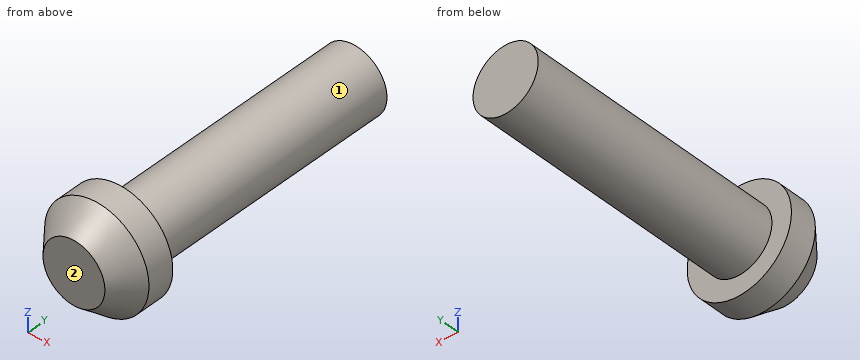
```python
from build123d import *

# Parameters (mm, degrees)
F1_DEPTH = 15.875
F3_DEPTH = 3.175


with BuildPart() as f1:
    # F0 (on Front) → F1 (new body)
    with BuildSketch(Plane.XZ):
        with BuildLine():
            ThreePointArc((-1.984375, 0), (0, -1.984375), (1.984375, 0))
            ThreePointArc((1.984375, 0), (0, 1.984375), (-1.984375, 0))
        make_face()
    extrude(amount=F1_DEPTH)

    # F2 (on face) → F3 (join)
    with BuildSketch(Plane.XZ.offset(15.875)):
        with BuildLine():
            ThreePointArc((3.175, 0), (0, 3.175), (-3.175, 0))
            ThreePointArc((-3.175, 0), (0, -3.175), (3.175, 0))
        make_face()
        with BuildLine():
            ThreePointArc((1.984375, 0), (0, -1.984375), (-1.984375, 0))
            ThreePointArc((-1.984375, 0), (0, 1.984375), (1.984375, 0))
        make_face(mode=Mode.SUBTRACT)
        with BuildLine():
            ThreePointArc((1.984375, 0), (0, 1.984375), (-1.984375, 0))
            ThreePointArc((-1.984375, 0), (0, -1.984375), (1.984375, 0))
        make_face()
    extrude(amount=F3_DEPTH)

    # F4 (on Right) → F5 (revolve, cut)
    with BuildSketch(Plane.YZ):
        Polygon((-19.8592845504, 1.2116890307), (-16.6845522668, 3.8504265809), (-19.8592845504, 3.8091964072), align=None)
    revolve(axis=Axis((0, -12.0745478198, 0), (0, -1, 0)), mode=Mode.SUBTRACT)


solid = f1.part
```
Check sheet for the modelled part. Datum: model origin and axes. Units: mm. Face numbers are marked on the shaded views. A direction names the side the tool comes from. Give positions to 0.01 mm unless a question says otherwise; leave off trailing zeros. Order: outer loops, then holes, each group sorted by start corner. A loop starts at its lowest first (then second) coordinate and runs counter-clockwise, first axis right, second up. Notation, with made-up numbers: M 4.5,42.5 L 56.5,42.5 A17 ccw 56.5,72.5 Z; hole C 18,16.25 d10. An arc over 180 degrees is marked long. Answer in a Markdown table with one row per item.
1) Thickness scan on L1, parallel to Z at x = 0, y = -4.75; L2, parallel to Z at x = 1.75, y = -5.5; L3, parallel to X at y = -14.5, z = -0.5. Record the ranges inside material, lowest first. Write a range as [from, to].
Filled sheet:
| item | result |
|---|---|
| L1 | z = [-1.98, 1.98] |
| L2 | z = [-0.94, 0.94] |
| L3 | x = [-1.92, 1.92] |
2) Cross-section at A-A, the plane x = 0. Enter the section's corners in (y, z) (3 decimals), plus the area to 3 significant figures.
Filled sheet:
| item | result |
|---|---|
| outline | M -19.05,-1.884 L -17.497,-3.175 L -15.875,-3.175 L -15.875,-1.984 L 0,-1.984 L 0,1.984 L -15.875,1.984 L -15.875,3.175 L -17.497,3.175 L -19.05,1.884 Z |
| area | 81.2 mm2 |
3) Cross-section at B-B, the plane z = 0. Enter the section's corners in (x, y) (3 decimals).
Filled sheet:
| item | result |
|---|---|
| outline | M -3.175,-17.497 L -1.884,-19.05 L 1.884,-19.05 L 3.175,-17.497 L 3.175,-15.875 L 1.984,-15.875 L 1.984,0 L -1.984,0 L -1.984,-15.875 L -3.175,-15.875 Z |
4) Gauge pin test, flat end, axial feed: P1, Ø1, axis at x = -2, y = -11, coming from the -Z side. Record the tip position at first contact, or that the pin passes through.
Filled sheet:
| item | result |
|---|---|
| P1 | stops at z = -1.3 |
5) Access from +Z, -Z, +X, -X, +Y, -Y to the whole of each face (thin tool, end or side, straight path). Record for the marked faces 1 and 2.
Filled sheet:
| item | result |
|---|---|
| face 1 | +Y |
| face 2 | +Z, -Z, +X, -X, -Y |
6) Cross-section at C-C, the plane y = -2. Enter the section's corners in (x, z).
Filled sheet:
| item | result |
|---|---|
| outline | C 0,0 d3.97 |
